Source: three-view drawing plus pictorial views. Frame: mm from the lowest corner of the part. A direction names the side the tool comes from. Give positions to 0.01 mm unless a question says otherwise; leave off trailing zeros. Order: outer loops, then holes, each group sorted by start corner. A loop starts at its lowest first (then second) coordinate and runs counter-clockwise, first axis right, second up. Notation, with made-up numbers: (80.25, 13) -> (87.25, 13) arc R8 cw to (87.25, 25) -> close; hole circle Ø6 at (44.5, 82.25). An arc over 180 degrees is marked (long way). Answer in a Markdown table with one row per item.
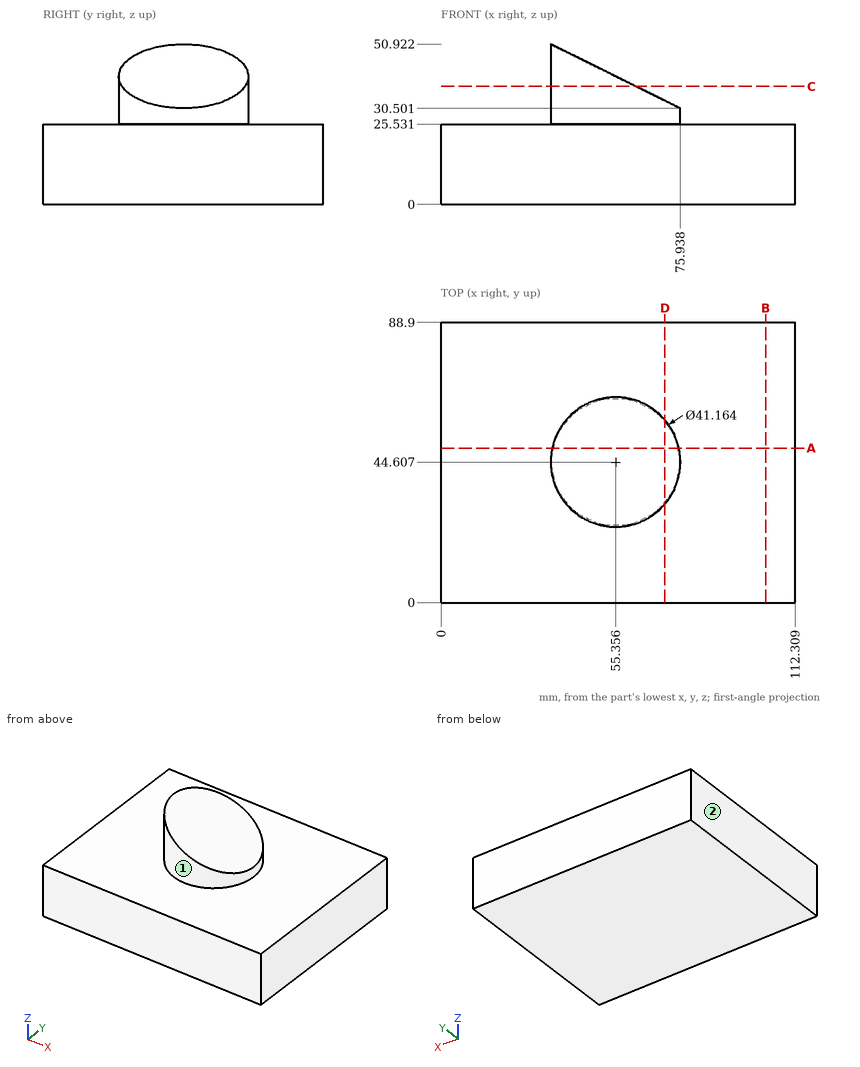
(1) Ray query, probe 1 along Z at (x, y) = (95, 25); probe 2 along X at (y, z) = (60, 40); probe 3 along Y at (x, z) = (42, 32). Return the intervals inside material, ascending.
A:
| item | result |
|---|---|
| probe 1 | z = 0 to 25.53 |
| probe 2 | x = 41.69 to 56.79 |
| probe 3 | y = 28.95 to 60.27 |
(2) Access query for the marked faces 1 and 2. Directions: +Z, -Z, +X, -X, +Y, -Y. A direction counts if a zero-diameter tool reaches every point of the face in a straight line with its end or side. Return the directions, or none.
A:
| item | result |
|---|---|
| face 1 | +Z |
| face 2 | +Z, -Z, -X, +Y, -Y |
(3) Section query D-D (x = 71). Return the cut outline in (y, z), plus the area to 3 significant figures.
A:
| item | result |
|---|---|
| outline | (0, 0) -> (88.9, 0) -> (88.9, 25.53) -> (57.98, 25.53) -> (57.98, 32.95) -> (31.23, 32.95) -> (31.23, 25.53) -> (0, 25.53) -> close |
| area | 2,470 mm^2 |
(4) Section query A-A (y = 49). Return the cut outline in (x, z).
A:
| item | result |
|---|---|
| outline | (0, 0) -> (112.31, 0) -> (112.31, 25.53) -> (75.46, 25.53) -> (75.46, 30.74) -> (35.25, 50.69) -> (35.25, 25.53) -> (0, 25.53) -> close |
(5) First-contact query: pin 1 Ø1.5 at (x, z) = (32, 20) entering from -Y; pin 2 Ø3 at (y, z) = (42, 42) entering from -X; pin 3 Ø4 at (x, y) = (90.5, 25) entering from +Z; pin 4 Ø2 at (x, y) = (42.5, 28.5) entering from +Z. Flat tips, straight axial feed; report the tip coordinate or a pass-through.
A:
| item | result |
|---|---|
| pin 1 | stops at y = 0 |
| pin 2 | stops at x = 34.8 |
| pin 3 | stops at z = 25.53 |
| pin 4 | stops at z = 47.46 |
(6) Section query B-B (x = 103). Return the cut outline in (y, z), plus the area to 3 significant figures.
A:
| item | result |
|---|---|
| outline | (0, 0) -> (88.9, 0) -> (88.9, 25.53) -> (0, 25.53) -> close |
| area | 2,270 mm^2 |
(7) Section query C-C (z = 37.5). Return the cut outline in (x, y).
A:
| item | result |
|---|---|
| outline | (61.83, 25.07) -> (61.83, 64.14) arc R20.58 ccw (long way) to start |
